Could you check a few things on this model? Use its own coordinates, in mm. Face numbers are marked on the shaded views. A direction names the side the tool comes from. Round coordinates to 2 decimals unless told otherwise and drop trailing zeros. Loops run counter-clockwise (first coordinate to the right, second up) from the corner with the lowest first, then second, coordinate; pieces in that order, holes last. Notation, with made-up numbers: (68, -31.5) - (73, -31.5) arc R16 ccw to (73, -14.5) - close; hole circle Ø9 at (69, 11). An arc over 180 degrees is marked (long way). Use one line per item in the form item = value.
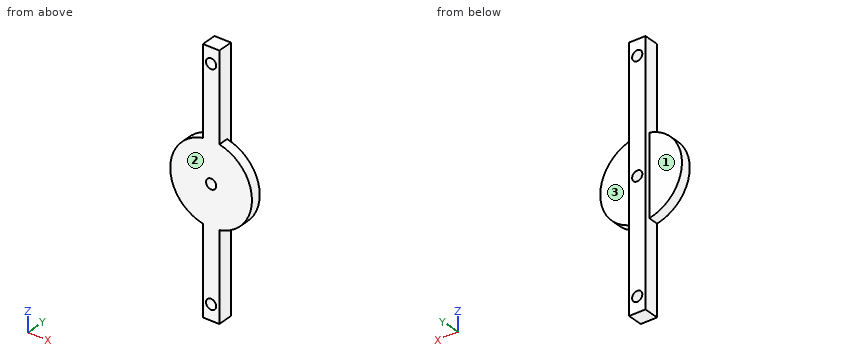
```python
from build123d import *

# Parameters (mm, degrees)
CROQUIS1_W                 = 16.099128824
CROQUIS1_H                 = 250
SALIENTE_EXTRUIR1_DEPTH    = 15
CROQUIS2_R                 = 40
SALIENTE_EXTRUIR2_DEPTH    = 10
CORTAR_EXTRUIR1_DEPTH      = 133.098448136
CORTAR_EXTRUIR1_DEPTH_BACK = 133.098448136
CROQUIS3_R                 = 5


with BuildPart() as part:
    # Croquis1 → Saliente-Extruir1 (new body)
    with BuildSketch(Plane(origin=(0, 0, 0), x_dir=(1, 0, 0), z_dir=(0, 1, 0))):
        Rectangle(CROQUIS1_W, CROQUIS1_H)
    extrude(amount=SALIENTE_EXTRUIR1_DEPTH)

    # Croquis2 → Saliente-Extruir2 (add)
    with BuildSketch(Plane(origin=(0, 0, 0), x_dir=(1, 0, 0), z_dir=(0, 1, 0))):
        Circle(CROQUIS2_R)
    extrude(amount=SALIENTE_EXTRUIR2_DEPTH)

    # Croquis3 → Cortar-Extruir1 (cut, two sides: drawn at the far end of the back side and taken through both)
    with BuildSketch(Plane(origin=(0, 0, 0), x_dir=(1, 0, 0), z_dir=(0, 1, 0)).offset(-CORTAR_EXTRUIR1_DEPTH_BACK)):
        with Locations(Location((0, 0, 0), (0, 0, 270))):
            Circle(CROQUIS3_R)
        with Locations(Location((0, 110, 0), (0, 0, 270))):
            Circle(CROQUIS3_R)
        with Locations(Location((0, -110, 0), (0, 0, 90))):
            Circle(CROQUIS3_R)
    extrude(amount=CORTAR_EXTRUIR1_DEPTH + CORTAR_EXTRUIR1_DEPTH_BACK, mode=Mode.SUBTRACT)


solid = part.part
```
1. If we section it at D-D, the plane z = -110: Write out the boundary of the cut face in (x, y).
Solution:
outline = (-8.05, 0) - (-5, 0) - (-5, 15) - (-8.05, 15) - close; (5, 0) - (8.05, 0) - (8.05, 15) - (5, 15) - close
2. If we section it at B-B, the plane y = 5.25: Write out the boundary of the cut face in (x, z).
Solution:
outline = (-8.05, -125) - (8.05, -125) - (8.05, -39.18) arc R40 ccw to (8.05, 39.18) - (8.05, 125) - (-8.05, 125) - (-8.05, 39.18) arc R40 ccw to (-8.05, -39.18) - close; hole circle Ø10 at (0, -110); hole circle Ø10 at (0, 0); hole circle Ø10 at (0, 110)
3. For P1, Ø7.5, axis at y = 8, z = -24, coming from the -X side; P2, Ø1.5, axis at y = 5.5, z = 52.5, coming from the -X side; P3, Ø13, axis at x = 0, z = 110, coming from the -Y side; P4, Ø4, axis at x = -19, y = 10.5, coming from the -Z side, each with a flat end and sliding along its axis, tell me the tip position at first contact or that it passes through.
Solution:
P1 = -34.5
P2 = -8.05
P3 = 0
P4 = -36.18
4. Please list where these lines run through material, in increasing order: line 1 along X through (y, z) = (11, -110); line 2 along Z through (x, y) = (-2, 7); line 3 along X through (y, z) = (4.25, 76.5).
Solution:
line_1 = -8.05 to -5, 5 to 8.05
line_2 = -125 to -114.58, -105.42 to -4.58, 4.58 to 105.42, 114.58 to 125
line_3 = -8.05 to 8.05
5. If we section it at A-A, the plane z = 0: Write out the boundary of the cut face in (x, y), plus the area to 3 significant figures.
Solution:
outline = (-40, 0) - (-5, 0) - (-5, 15) - (-8.05, 15) - (-8.05, 10) - (-40, 10) - close; (5, 0) - (40, 0) - (40, 10) - (8.05, 10) - (8.05, 15) - (5, 15) - close
area = 730 mm^2
6. On a 3-axis mill with a long thin cutter (end or side, diameter ignored), from which of +Z, -Z, +X, -X, +Y, -Y can I reach the whole of each face in a straight line? I mean the marked faces 1, 2 and 3. Say none if no direction works.
Solution:
face_1 = +Z, -Z, -X, +Y
face_2 = +Z, -Z, +X, -X, -Y
face_3 = +Z, -Z, +X, +Y
7. If we section it at C-C, the plane x = 0: Write out the boundary of the cut face in (y, z), plus the area to 3 significant figures.
Solution:
outline = (0, -125) - (15, -125) - (15, -115) - (0, -115) - close; (0, -105) - (15, -105) - (15, -5) - (0, -5) - close; (0, 5) - (15, 5) - (15, 105) - (0, 105) - close; (0, 115) - (15, 115) - (15, 125) - (0, 125) - close
area = 3,300 mm^2
